Here's how the part is built. I have some questions about the finished solid (model axes, mm). A direction names the side the tool comes from. Round coordinates to 2 decimals unless told otherwise and drop trailing zeros. Write each loop counter-clockwise with the first axis right and the second up, starting at its lowest first coordinate (ties: lowest second). Pieces come first, ordered by that corner, then holes. Notation, with made-up numbers: M -3,54 L 54,54 A26 ccw 54,71 Z; hole C 54,40 d8. An arc over 180 degrees is marked long. Use one line per item in the form item = value. Start each with the question number.
Q1. For faces 4 (the face through (35.195, -0.531, 0.986)), 5 (the face through (105, 15, 2)), which set-ups out of +Z, -Z, +X, -X, +Y, -Y let a thin tool reach every point of the face, with its end or its side?
Q2. I want a section at A-A on x = 166. List the corners of the cut face in (y, z) for me.
Q3. I want a section at D-D on x = 210. List the corners of the cut face in (y, z) for me, and give its area (3 significant figures).
Q4. I'm going to push flat-ended pins straight in: pin 1 Ø1 at (x, z) = (162, 1) entering from -Y; pin 2 Ø8 at (x, y) = (196.5, -10.5) entering from +Z; pin 3 Ø0.6 at (x, z) = (170.5, 1) entering from +Y. Where does each tip first touch, or does it pass through?
Q5. I want a section at C-C on x = 253.5. List the corners of the cut face in (y, z) for me, and give its area (3 significant figures).
Q6. I need wall thicknesses on line 1 along Y through (x, z) = (77.5, 0.15); line 2 along Y through (x, z) = (98, 0.2); line 3 along Y through (x, z) = (62.5, 0.3). Which ranges of each line are inside material? Lowest first, please. Write a range as from..to.
Q7. I want a section at B-B on z = 0.9. State how many separate pieces and enclosed holes the cut face has, and give its area (3 significant figures).
Q8. We'd pull the mould along Y, two halves only. Please class faces 1 (the face through (55.29, -2.56, 0.99)), 2 (the face through (204.02, -0.42, 0.99)), 3 (the face through (105, 15, 0)): +Y half, -Y half, draft (parallel to the pull), parting line (faces both ways), or undercut.
```python
from build123d import *

# Parameters (mm, degrees)
SKETCH_1_W      = 135
SKETCH_1_H      = 60.000000048
SKETCH_1_W_2    = 50
SKETCH_1_H_2    = 2
SKETCH_1_R      = 2.5
SKETCH_1_W_3    = 45
SKETCH_1_H_3    = 2.000000262
SKETCH_1_W_4    = 70.000000056
EXTRUDE_1_DEPTH = 2


with BuildPart() as part:
    # 草图1 → 凸台-拉伸1 (new body)
    # profile 1 of 5: a face of its own
    with BuildSketch(Plane.XY):
        with Locations((67.5, -2.86e-07)):
            Rectangle(SKETCH_1_W, SKETCH_1_H)
        with BuildLine():
            ThreePointArc((68.064332648, 0.863431574), (67.5, 0.944700571), (66.935667352, 0.863431574))
            Line((66.935667352, 0.863431574), (43.323685411, -6.081268997))
            ThreePointArc((43.323685411, -6.081268997), (41.908439567, -8.285077177), (43.888018059, -10))
            Line((43.888018059, -10), (91.111981941, -10))
            ThreePointArc((91.111981941, -10), (93.091560433, -8.285077177), (91.676314589, -6.081268997))
            Line((91.676314589, -6.081268997), (68.064332648, 0.863431574))
        make_face(mode=Mode.SUBTRACT)
        with BuildLine():
            ThreePointArc((66.935667352, 9.136568426), (67.5, 9.055299429), (68.064332648, 9.136568426))
            Line((68.064332648, 9.136568426), (91.676314589, 16.081268997))
            ThreePointArc((91.676314589, 16.081268997), (93.091560433, 18.285077177), (91.111981941, 20))
            Line((91.111981941, 20), (43.888018059, 20))
            ThreePointArc((43.888018059, 20), (41.908439567, 18.285077177), (43.323685411, 16.081268997))
            Line((43.323685411, 16.081268997), (66.935667352, 9.136568426))
        make_face(mode=Mode.SUBTRACT)
        with Locations((65, -19)):
            Rectangle(SKETCH_1_W_2, SKETCH_1_H_2, mode=Mode.SUBTRACT)
        with BuildLine():
            Line((47.476314589, 3.081268997), (22.564332648, -4.245784515))
            ThreePointArc((22.564332648, -4.245784515), (20.80180663, -3.928406892), (20, -2.327053512))
            Line((20, -2.327053512), (20, 12.327053512))
            ThreePointArc((20, 12.327053512), (20.80180663, 13.928406892), (22.564332648, 14.245784515))
            Line((22.564332648, 14.245784515), (47.476314589, 6.918731003))
            ThreePointArc((47.476314589, 6.918731003), (48.911981941, 5), (47.476314589, 3.081268997))
        make_face(mode=Mode.SUBTRACT)
        with BuildLine():
            Line((87.523685411, 3.081268997), (112.435667352, -4.245784515))
            ThreePointArc((112.435667352, -4.245784515), (114.19819337, -3.928406892), (115, -2.327053512))
            Line((115, -2.327053512), (115, 12.327053512))
            ThreePointArc((115, 12.327053512), (114.19819337, 13.928406892), (112.435667352, 14.245784515))
            Line((112.435667352, 14.245784515), (87.523685411, 6.918731003))
            ThreePointArc((87.523685411, 6.918731003), (86.088018059, 5), (87.523685411, 3.081268997))
        make_face(mode=Mode.SUBTRACT)
    # profile 2 of 5: a face of its own
    with BuildSketch(Plane.XY):
        Polygon((135, -10), (135, -30.00000031), (275.000000112, 29.999999738), (205.000000056, 29.999999738), (135, 29.999999738), (135, 10), (137, 10), (137, -10), align=None)
        with BuildLine():
            Line((171.04398986, -3.83829006), (147.787838597, -13.80521203))
            ThreePointArc((147.787838597, -13.80521203), (145.899017983, -13.636604154), (145, -11.96692197))
            Line((145, -11.96692197), (145, -2))
            ThreePointArc((145, -2), (145.585786438, -0.585786438), (147, 0))
            Line((147, 0), (170.256151263, 0))
            ThreePointArc((170.256151263, 0), (172.215306708, -1.597868255), (171.04398986, -3.83829006))
        make_face(mode=Mode.SUBTRACT)
        with Locations((150.760493498, 16.868933163)):
            Circle(SKETCH_1_R, mode=Mode.SUBTRACT)
        Polygon((218.565739708, 14.508933163), (218.565739708, 16.868933163), (218.565739708, 23.287933163), (220.565739708, 23.287933163), (220.565739708, 14.508933163), align=None, mode=Mode.SUBTRACT)
    # profile 3 of 5: a face of its own
    with BuildSketch(Plane.XY):
        with Locations((112.5, 30.999999869)):
            Rectangle(SKETCH_1_W_3, SKETCH_1_H_3)
    # profile 4 of 5: a face of its own
    with BuildSketch(Plane.XY):
        with Locations((25, 30.999999869)):
            Rectangle(SKETCH_1_W_2, SKETCH_1_H_3)
    # profile 5 of 5: a face of its own
    with BuildSketch(Plane.XY):
        with Locations((240.000000084, 30.999999869)):
            Rectangle(SKETCH_1_W_4, SKETCH_1_H_3)
    extrude(amount=EXTRUDE_1_DEPTH)


solid = part.part
```
Reported:
q1.face_4 = +Z, -Z
q1.face_5 = +Z, +X, -X, +Y, -Y
q2.outline = M -16.71,0 L -6,0 L -6,2 L -16.71,2 Z; M 0,0 L 30,0 L 30,2 L 0,2 Z
q3.outline = M 2.14,0 L 32,0 L 32,2 L 2.14,2 Z
q3.area = 59.7 mm^2
q4.pin_1 = -18.64
q4.pin_2 = through
q4.pin_3 = 30
q5.outline = M 20.79,0 L 32,0 L 32,2 L 20.79,2 Z
q5.area = 22.4 mm^2
q6.line_1 = -30..-20, -18..-10, -1.91..11.91, 20..30
q6.line_2 = -30..0, 10..32
q6.line_3 = -30..-20, -18..-10, -0.44..10.44, 20..30
q7.separate_pieces = 1
q7.enclosed_holes = 9
q7.area = 10,800 mm^2
q8.face_1 = undercut
q8.face_2 = -Y half
q8.face_3 = draft
